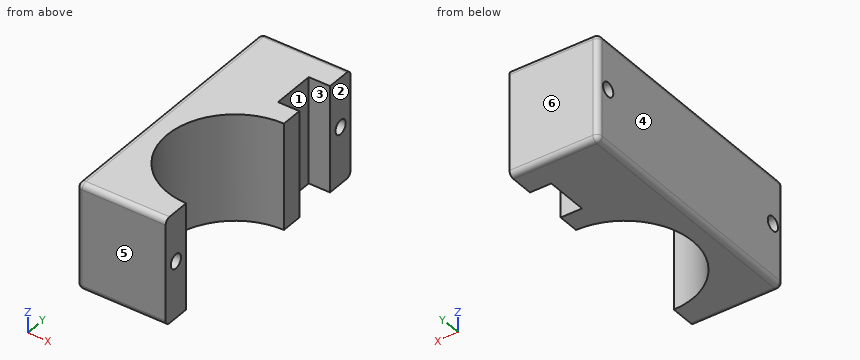
Autodesk Fusion 360 part; units mm, degrees
sketch "Esboço1" plane through (0, 0, 0) normal (0, 0, 1) x (1, 0, 0)
  line L0 (15, 50.1) -> (21, 50.1)
  line L1 (15, 62.1) -> (15, 50.1)
  line L2 (-4, -2.1) -> (-4, 70.1)
  line L3 (-4, -2.1) -> (21, -2.1)
  line L4 (21, 70.1) -> (21, 62.1)
  line L5 (21, 62.1) -> (15, 62.1)
  line L6 (21, 5.9) -> (21, -2.1)
  line L7 (21, 50.1) -> (21, 44.1)
  arc A0 (21, 44.1) -> (21, 5.9) centre (21, 25) ccw
  line L8 (-4, 70.1) -> (21, 70.1)
  dimension "d2" = 12
  dimension "d3" = 6
  dimension "d5" = 8
  dimension "d8" = 6
  dimension "d10" = 8
  dimension "d36" = 25
  dimension "d12" = 6
  dimension "d13" = 19.1
extrude "Extrusão1" add sketch "Esboço1" along normal blind 30
hole "Furo1" at (-4, 66.2367, 16) direction (1, 0, 0) diameter 4 depth 25 tip angle 180
hole "Furo2" at (-4, 1.9, 16) direction (1, 0, 0) diameter 4 depth 25 tip angle 180
fillet "Arredondamento1" radius 1.5 5 edges at (-4, 34, 30) (-4, -2.1, 15) (8.5, -2.1, 30) (8.5, -2.1, 0) (-4, 34, 0)
fillet "Arredondamento2" radius 1.5 5 edges at (9.25, 70.1, 30) (-3.5607, 70.1, 29.5607) (-4, 70.1, 15) (-3.5607, 70.1, 0.4393) (9.25, 70.1, 0)
Can you work these out from the model? Positions are in its coordinate system, mm. Face numbers are marked on the shaded views. A direction names the side the tool comes from. Round coordinates to 2 decimals unless told otherwise and drop trailing zeros. Loops run counter-clockwise (first coordinate to the right, second up) from the corner with the lowest first, then second, coordinate; pieces in that order, holes last.
Item 1: Will these pins go through, and if not, where does the flat tip stop? pin 1 Ø8 at (y, z) = (13, 6) entering from +X; pin 2 Ø2.5 at (y, z) = (1.9, 16) entering from +X.
Item 2: If we mould it in two halves opening along Y, with no side actions, what happens to the marked faces 3, 4, 5 and 6? For each: +Y half, -Y half, draft (parallel to the pull), parting line (faces both ways), or undercut.
Item 3: Suppose I cut it at D-D, the plane z = 20. Write out the boundary of the cut face in (x, y).
Item 4: Suppose I cut it at B-B, the plane x = 3.75. Write out the boundary of the cut face in (y, z), then the cut area to 3 significant figures.
Item 5: Suppose I cut it at C-C, the plane x = 16.25. Write out the boundary of the cut face in (y, z), then the cut area to 3 significant figures.
Item 6: Please list where these lines run through material, in increasing order: L1, parallel to Y at x = 10, z = 16; L2, parallel to Y at x = 16, z = 24.5; L3, parallel to Y at x = 13.25, z = 16.
Item 7: Which directions (+Z, -Z, +X, -X, +Y, -Y) give clear straight access to the entire face, cutting with the end or side of a thin tool? Please do the marked faces 1 and 2.
Item 8: Suppose I cut it at A-A, the plane y = 1.9. Write out the boundary of the cut face in (x, z), then the cut area to 3 significant figures.
Reported:
1. pin 1: stops at x = 10.57
1. pin 2: passes through
2. face 3: undercut
2. face 4: draft
2. face 5: -Y half
2. face 6: +Y half
3. outline: (-4, -0.6) arc R1.5 ccw to (-2.5, -2.1) - (21, -2.1) - (21, 5.9) arc R19.1 cw to (21, 44.1) - (21, 50.1) - (15, 50.1) - (15, 62.1) - (21, 62.1) - (21, 70.1) - (-2.5, 70.1) arc R1.5 ccw to (-4, 68.6) - close
4. outline: (-2.1, 1.5) arc R1.5 ccw to (-0.6, 0) - (16.8, 0) - (16.8, 30) - (-0.6, 30) arc R1.5 ccw to (-2.1, 28.5) - close; (33.2, 0) - (68.6, 0) arc R1.5 ccw to (70.1, 1.5) - (70.1, 28.5) arc R1.5 ccw to (68.6, 30) - (33.2, 30) - close; hole circle Ø4 at (1.9, 16); hole circle Ø4 at (66.24, 16)
4. area: 1,650 mm2
5. outline: (-2.1, 1.5) arc R1.5 ccw to (-0.6, 0) - (6.5, 0) - (6.5, 30) - (-0.6, 30) arc R1.5 ccw to (-2.1, 28.5) - close; (43.5, 0) - (50.1, 0) - (50.1, 30) - (43.5, 30) - close; (62.1, 0) - (68.6, 0) arc R1.5 ccw to (70.1, 1.5) - (70.1, 28.5) arc R1.5 ccw to (68.6, 30) - (62.1, 30) - close; hole circle Ø4 at (1.9, 16); hole circle Ø4 at (66.24, 16)
5. area: 669 mm2
6. L1: y = -2.1 to -0.1, 3.9 to 9.39, 40.61 to 64.24, 68.24 to 70.1
6. L2: y = -2.1 to 6.57, 43.43 to 50.1, 62.1 to 70.1
6. L3: y = -2.1 to -0.1, 3.9 to 7.54, 42.46 to 64.24, 68.24 to 70.1
7. face 1: +Z, -Z, +X
7. face 2: +Z, -Z, +X, +Y, -Y
8. outline: (-4, 1.5) arc R1.5 ccw to (-2.5, 0) - (21, 0) - (21, 14) - (-4, 14) - close; (-4, 18) - (21, 18) - (21, 30) - (-2.5, 30) arc R1.5 ccw to (-4, 28.5) - close
8. area: 649 mm2
